Can you work these out from the model? Positions are in its coordinate system, mm. Give positions to 0.01 mm unless a question says otherwise; leave off trailing zeros. Order: outer loops, then holes, each group sorted by start corner. A loop starts at its lowest first (then second) coordinate and runs counter-clockwise, first axis right, second up.
Item 1: I want a section at B-B, the plane y = 0.65. Write out the boundary of the cut face in (x, z) (1 decimal), then the cut area to 3 significant figures.
Item 2: I want a section at C-C, the plane x = 25.4. Write out the boundary of the cut face in (y, z).
Item 3: I want a section at A-A, the plane z = 1. Write out the boundary of the cut face in (x, y), then the cut area to 3 significant figures.
Item 4: If I drill on line 1 along Z through (x, y) = (0, 0.75); line 2 along X through (y, z) = (1.35, 24.5); line 3 along X through (y, z) = (1.15, 25.5), over which ranges is the centre line in solid material (lowest first)?
Item 5: I'm going to push flat-ended pins straight in: pin 1 Ø6.5 at (x, z) = (0, 50.8) entering from +Y; pin 2 Ø0.8 at (x, y) = (17.5, 0.5) entering from +Z. Where does each tip first touch, or does it pass through?
Item 6: I want a section at D-D, the plane z = 29. Write out the boundary of the cut face in (x, y).
Autodesk Inventor part; units mm, degrees
ref_plane "YZ Plane" through (0, 0, 0) normal (1, 0, 0) x (0, 1, 0)
ref_plane "XZ Plane" through (0, 0, 0) normal (0, 1, 0) x (-1, 0, 0)
ref_plane "XY Plane" through (0, 0, 0) normal (0, 0, 1) x (1, 0, 0)
sketch "main" plane through (0, 0, 0) normal (0, 0, 1) x (1, 0, 0)
  circle A0 centre (27.8145, 23.5161) radius 2.0955
  circle A1 centre (27.8145, -27.2839) radius 2.0955
  circle A2 centre (-22.9855, -27.2839) radius 2.0955
  arc A3 (-26.3531, -23.9163) -> (-22.9855, -32.0464) centre (-22.9855, -27.2839) ccw
  arc A4 (27.8145, -32.0464) -> (32.577, -27.2839) centre (27.8145, -27.2839) ccw
  arc A5 (32.577, 23.5161) -> (24.4469, 26.8837) centre (27.8145, 23.5161) ccw
  line L0 (32.577, 23.5161) -> (32.577, -27.2839)
  line L1 (27.8145, -32.0464) -> (-22.9855, -32.0464)
  line L2 (24.4469, 26.8837) -> (-26.3531, -23.9163)
  line L3 (-11.4879, -22.5214) -> (23.052, -22.5214)
  line L4 (23.052, -22.5214) -> (23.052, 12.0184)
  line L5 (23.052, 12.0184) -> (-11.4879, -22.5214)
  circle A6 centre (2.4145, -1.8839) radius 2.0955
  point P0 (11.2944, -10.7639)
  dimension "d3" = 4.191
  dimension "d4" = 4.191
  dimension "d5" = 4.191
  dimension "d7" = 9.525
  dimension "d8" = 4.191
  dimension "d9" = 4.7625
  dimension "d10" = 4.7625
  dimension "d11" = 4.7625
sketch "Sketch1" plane through (0, 0, 0) normal (0, 1, 0) x (-1, 0, 0)
  circle A0 centre (-25.4, 0) radius 2.0955
  circle A1 centre (0, 25.4) radius 2.0955
  circle A2 centre (0, 50.8) radius 2.0955
  circle A3 centre (0, 0) radius 2.0955
  circle A4 centre (-50.8, 0) radius 2.0955
  arc A5 (-54.1676, 3.3676) -> (-50.8, -4.7625) centre (-50.8, 0) ccw
  arc A6 (0, -4.7625) -> (4.7625, 0) centre (0, 0) ccw
  arc A7 (4.7625, 50.8) -> (-3.3676, 54.1676) centre (0, 50.8) ccw
  line L0 (4.7625, 50.8) -> (4.7625, 0)
  line L1 (0, -4.7625) -> (-50.8, -4.7625)
  line L2 (-3.3676, 54.1676) -> (-54.1676, 3.3676)
  line L3 (-39.3023, 4.7625) -> (-4.7625, 4.7625)
  line L4 (-4.7625, 4.7625) -> (-4.7625, 39.3023)
  line L5 (-4.7625, 39.3023) -> (-39.3023, 4.7625)
  circle A8 centre (-25.4, 25.4) radius 2.0955
  dimension "d2" = 4.191
  dimension "d6" = 4.191
extrude "Extrusion1" add sketch "Sketch1" along normal blind 1.5875
equation "\"BendRadius\" = Thickness"
equation "\"BendReliefWidth\" = Thickness"
equation "\"BendReliefDepth\" = 0.5 * Thickness"
equation "\"CornerReliefSize\" = 4 * Thickness"
equation "\"MinimumRemnant\" = 2 * Thickness"
equation "\"TransitionRadius\" = BendRadius"
equation "\"JacobiRadiusSize\" = BendRadius"
equation "\"GapSize\" = Thickness"
properties part number "Arm Triangle Gusset" material "Acetal Resin, White"
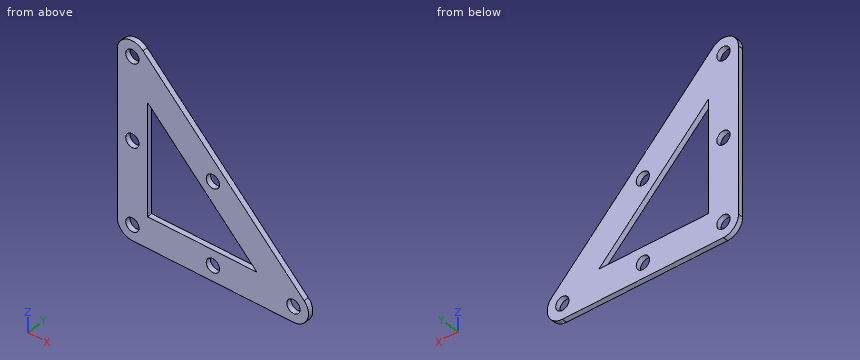
Results list:
1. outline: (-4.8, 0) arc R4.8 ccw to (0, -4.8) - (50.8, -4.8) arc R4.8 ccw to (54.2, 3.4) - (3.4, 54.2) arc R4.8 ccw to (-4.8, 50.8) - close; hole circle Ø4.2 at (0, 0); hole circle Ø4.2 at (0, 25.4); hole circle Ø4.2 at (0, 50.8); hole (4.8, 4.8) - (39.3, 4.8) - (4.8, 39.3) - close; hole circle Ø4.2 at (25.4, 0); hole circle Ø4.2 at (25.4, 25.4); hole circle Ø4.2 at (50.8, 0)
1. area: 1,510 mm2
2. outline: (0, -4.76) - (1.59, -4.76) - (1.59, -2.1) - (0, -2.1) - close; (0, 2.1) - (1.59, 2.1) - (1.59, 4.76) - (0, 4.76) - close; (0, 18.66) - (1.59, 18.66) - (1.59, 23.3) - (0, 23.3) - close; (0, 27.5) - (1.59, 27.5) - (1.59, 32.14) - (0, 32.14) - close
3. outline: (-4.76, 0) - (-1.84, 0) - (-1.84, 1.59) - (-4.76, 1.59) - close; (1.84, 0) - (23.56, 0) - (23.56, 1.59) - (1.84, 1.59) - close; (27.24, 0) - (48.96, 0) - (48.96, 1.59) - (27.24, 1.59) - close; (52.64, 0) - (55.46, 0) - (55.46, 1.59) - (52.64, 1.59) - close
3. area: 78.1 mm2
4. line 1: z = -4.76 to -2.1, 2.1 to 23.3, 27.5 to 48.7, 52.9 to 55.56
4. line 2: x = -4.76 to -1.89, 1.89 to 4.76, 19.56 to 23.51, 27.29 to 33.04
4. line 3: x = -4.76 to -2.09, 2.09 to 4.76, 18.56 to 23.31, 27.49 to 32.04
5. pin 1: stops at y = 1.59
5. pin 2: stops at z = 40.44
6. outline: (-4.76, 0) - (4.76, 0) - (4.76, 1.59) - (-4.76, 1.59) - close; (15.06, 0) - (28.54, 0) - (28.54, 1.59) - (15.06, 1.59) - close
